Part model, mm, in its own coordinate system. Face numbers are marked on the shaded views. A direction names the side the tool comes from. Coordinates: 2 decimals unless noted, no trailing zeros. Order: outer loops, then holes, each group sorted by start corner. A loop starts at its lowest first (then second) coordinate and runs counter-clockwise, first axis right, second up. Notation, with made-up numbers: (-7.5, 19.25) - (50.5, 19.25) arc R33 ccw to (50.5, 52.25) - close; hole circle Ø1 at (52.5, 13.25). An arc over 180 degrees is marked (long way). Use a Markdown table: item, result. Add a question column.
1) Saw through at B-B on x = 29. List the corners of the cut face in (y, z).
2) Wall check: L1, parallel to Z at x = 15.5, y = 4.5; L2, parallel to Z at x = -14.5, y = 0.3; L3, parallel to X at y = 1.9, z = 26.5 (3 decimals). Give the ranges that are in metal, low to high. Write a range as [from, to].
3) Tool access for the marked faces 1, 2 and 3: list every direction of +Z, -Z, +X, -X, +Y, -Y with a clear straight run to the whole face (end or side of a thin tool).
4) Saw through at D-D on x = 2. List the corners of the cut face in (y, z).
5) Saw through at C-C on y = 1.65. List the corners of the cut face in (x, z) (1 decimal), then the cut area to 3 significant figures.
6) Saw through at A-A on z = -18.5. List the corners of the cut face in (x, y) (3 decimals), then the cut area to 3 significant figures.
7) Drop flat-ended pins along their axis: P1, Ø1.8, axis at y = 4.5, z = -28.5, coming from the +X side (3 decimals); P2, Ø3, axis at x = 28.26, z = 13.87, coming from the -Y side; P3, Ø1.8, axis at x = -26, y = 3.5, coming from the +Z side. Give the stop position or say it passes through.
```python
from build123d import *

# Parameters (mm, degrees)
BOSS_EXTRUDE1_DEPTH = 5.842
SKETCH2_R           = 1.778
CUT_EXTRUDE1_DEPTH  = 43.811518376
SKETCH3_W           = 5.08
SKETCH3_H           = 50.995072
BOSS_EXTRUDE2_DEPTH = 5.842
SKETCH4_R           = 1.5875
CUT_EXTRUDE2_DEPTH  = 47.356817252


with BuildPart() as part:
    # Sketch1 → Boss-Extrude1 (new body)
    with BuildSketch(Plane(origin=(0, 0, 0), x_dir=(1, 0, 0), z_dir=(0, 1, 0))):
        Polygon((22.325, -31.339536), (9.425, -31.339536), (9.425, -25.497536), (-9.425, -25.497536), (-9.425, -31.339536), (-22.325, -31.339536), (-22.325, -25.497536), (-28.575, -25.497536), (-28.575, 25.497536), (-22.325, 25.497536), (-22.325, 31.339536), (-9.425, 31.339536), (-9.425, 25.497536), (9.425, 25.497536), (9.425, 31.339536), (22.325, 31.339536), (22.325, 25.497536), (28.575, 25.497536), (28.575, -25.497536), (22.325, -25.497536), align=None)
    extrude(amount=BOSS_EXTRUDE1_DEPTH)

    # Sketch2 → Cut-Extrude1 (cut, through all)
    with BuildSketch(Plane(origin=(0, 5.842, 0), x_dir=(1, 0, 0), z_dir=(0, 1, 0))):
        with Locations(Location((-15.875, 28.418536, 0), (0, 0, 270))):
            Circle(SKETCH2_R)
        with Locations(Location((-15.875, -28.418536, 0), (0, 0, 270))):
            Circle(SKETCH2_R)
        with Locations(Location((15.875, 28.418536, 0), (0, 0, 90))):
            Circle(SKETCH2_R)
        with Locations(Location((15.875, -28.418536, 0), (0, 0, 90))):
            Circle(SKETCH2_R)
    extrude(amount=-CUT_EXTRUDE1_DEPTH, mode=Mode.SUBTRACT)

    # Sketch3 → Boss-Extrude2 (add)
    with BuildSketch(Plane(origin=(0, 5.842, 0), x_dir=(1, 0, 0), z_dir=(0, 1, 0))):
        with Locations((31.115, 0)):
            Rectangle(SKETCH3_W, SKETCH3_H)
    extrude(amount=-BOSS_EXTRUDE2_DEPTH)

    # Sketch4 → Cut-Extrude2 (cut, through all)
    with BuildSketch(Plane(origin=(0, 0, 0), x_dir=(-1, 0, 0), z_dir=(0, -1, 0))):
        with Locations(Location((23.8125, 19.147536, 0), (0, 0, 90))):
            Circle(SKETCH4_R)
        with Locations(Location((-28.2575, 14.067536, 0), (0, 0, 90))):
            Circle(SKETCH4_R)
        with Locations(Location((-28.2575, -13.872464, 0), (0, 0, 90))):
            Circle(SKETCH4_R)
    extrude(amount=-CUT_EXTRUDE2_DEPTH, mode=Mode.SUBTRACT)


solid = part.part
```
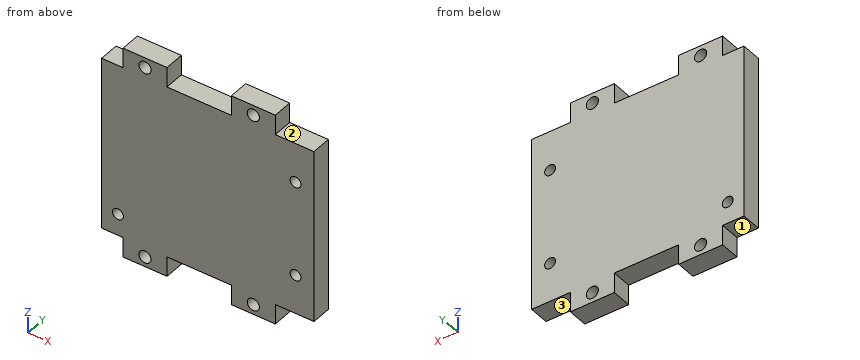
Results are:
| question | item | result |
|---|---|---|
| 1 | outline | (0, -25.5) - (5.84, -25.5) - (5.84, -15.47) - (0, -15.47) - close; (0, -12.66) - (5.84, -12.66) - (5.84, 12.47) - (0, 12.47) - close; (0, 15.28) - (5.84, 15.28) - (5.84, 25.5) - (0, 25.5) - close |
| 2 | L1 | [-31.34, -30.16], [-26.68, 26.68], [30.16, 31.34] |
| 2 | L2 | [-31.34, -29.55], [-27.29, 27.29], [29.55, 31.34] |
| 2 | L3 | [-22.325, -9.425], [9.425, 22.325] |
| 3 | face 1 | -Z, -X, +Y, -Y |
| 3 | face 2 | +Z, +X, +Y, -Y |
| 3 | face 3 | -Z, +X, +Y, -Y |
| 4 | outline | (0, -25.5) - (5.84, -25.5) - (5.84, 25.5) - (0, 25.5) - close |
| 5 | outline | (-28.6, -25.5) - (-22.3, -25.5) - (-22.3, -31.3) - (-9.4, -31.3) - (-9.4, -25.5) - (9.4, -25.5) - (9.4, -31.3) - (22.3, -31.3) - (22.3, -25.5) - (33.7, -25.5) - (33.7, 25.5) - (22.3, 25.5) - (22.3, 31.3) - (9.4, 31.3) - (9.4, 25.5) - (-9.4, 25.5) - (-9.4, 31.3) - (-22.3, 31.3) - (-22.3, 25.5) - (-28.6, 25.5) - close; hole circle Ø3.2 at (-23.8, -19.1); hole circle Ø3.6 at (-15.9, -28.4); hole circle Ø3.6 at (-15.9, 28.4); hole circle Ø3.6 at (15.9, -28.4); hole circle Ø3.6 at (15.9, 28.4); hole circle Ø3.2 at (28.3, -14.1); hole circle Ø3.2 at (28.3, 13.9) |
| 5 | area | 3,410 mm2 |
| 6 | outline | (-28.575, 0) - (-25.262, 0) - (-25.262, 5.842) - (-28.575, 5.842) - close; (-22.363, 0) - (33.655, 0) - (33.655, 5.842) - (-22.363, 5.842) - close |
| 6 | area | 347 mm2 |
| 7 | P1 | x = 22.325 |
| 7 | P2 | through |
| 7 | P3 | z = 25.5 |
